Input: part model. Units: mm. Frame: model coordinates. A direction names the side the tool comes from. Coordinates: 2 decimals unless noted, no trailing zeros. Order: outer loops, then holes, each group sorted by start corner. A loop starts at its lowest first (then second) coordinate and runs counter-clockwise, first axis right, second up.
from build123d import *

# Parameters (mm, degrees)
SKETCH1_R           = 6.35
BOSS_EXTRUDE1_DEPTH = 400.05
SKETCH1_3_R         = 25.4
SKETCH1_3_R_2       = 6.35
BOSS_EXTRUDE2_DEPTH = 381


with BuildPart() as part:
    # Sketch1 → Boss-Extrude1 (new, symmetric)
    with BuildSketch(Plane.XY):
        with Locations(Location((0, 0, 0), (0, 0, 180))):
            Circle(SKETCH1_R)
    extrude(amount=BOSS_EXTRUDE1_DEPTH, both=True)

    # Sketch1_3 → Boss-Extrude2 (add, symmetric)
    with BuildSketch(Plane.XY):
        Circle(SKETCH1_3_R)
        with Locations(Location((0, 0, 0), (0, 0, 180))):
            Circle(SKETCH1_3_R_2, mode=Mode.SUBTRACT)
    extrude(amount=BOSS_EXTRUDE2_DEPTH, both=True)


solid = part.part
Item 1: Cut plane B-B on y = -18. Return loops of the section in (x, z), then the cut area to 3 significant figures.
Response values:
outline: (-17.92, -381) - (17.92, -381) - (17.92, 381) - (-17.92, 381) - close
area: 27,300 mm2
Item 2: Pin query (flat end, axial travel): pin 1 Ø4 at (x, y) = (9, 20) entering from +Z; pin 2 Ø6 at (x, z) = (12.5, 90) entering from -Y; pin 3 Ø8 at (y, z) = (-4.5, 213) entering from +X. Return the tip coordinate at first contact, or that it passes through.
Response values:
pin 1: stops at z = 381
pin 2: stops at y = -23.56
pin 3: stops at x = 25.4
Item 3: Cut plane A-A on z = -254. Return loops of the section in (x, y).
Response values:
outline: circle Ø50.8 at (0, 0)
Item 4: Ray query, probe 1 along X at (y, z) = (-2, 193.5); probe 2 along Z at (x, y) = (-2, 12); probe 3 along Y at (x, z) = (1.5, 291). Return the intervals inside material, ascending.
Response values:
probe 1: x = -25.32 to 25.32
probe 2: z = -381 to 381
probe 3: y = -25.36 to 25.36
Item 5: Cut plane C-C on x = -15. Return loops of the section in (y, z).
Response values:
outline: (-20.5, -381) - (20.5, -381) - (20.5, 381) - (-20.5, 381) - close
Item 6: Access query for faces 1 (the face through (-2.93, 5.634, 390.658)), 2 (the face through (0, 0, -400.05)), 3 (the face through (-2.93, 5.634, -390.392)). Directions: +Z, -Z, +X, -X, +Y, -Y. A direction counts if a zero-diameter tool reaches every point of the face in a straight line with its end or side. Return the directions, or none.
Response values:
face 1: +Z
face 2: -Z, +X, -X, +Y, -Y
face 3: -Z
